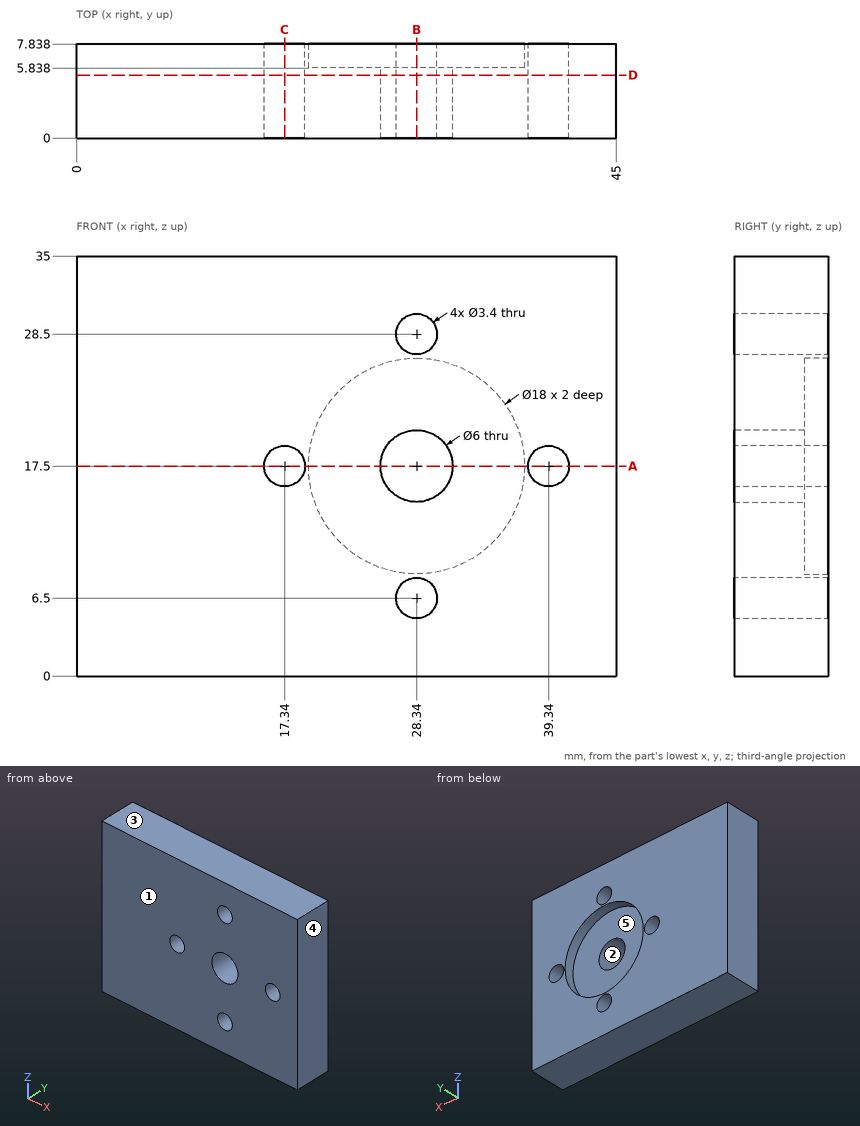
Geometry: see drawing. Coordinates: mm, zero at the bounding-box minimum. A direction names the side the tool comes from. Give positions to 0.01 mm unless a question says otherwise; leave off trailing zeros. Loops run counter-clockwise (first coordinate to the right, second up) from the corner with the lowest first, then second, coordinate; pieces in that order, holes last. Notation, with made-up numbers: (-17.75, -23) -> (-7.75, -23) arc R37 cw to (-7.75, 15) -> close; hole circle Ø3 at (-12, 40.5). An arc over 180 degrees is marked (long way). Put each result on its own line as item: value.
1. Cut plane B-B (x = 28.34). Return the cut outline in (y, z).
Taken from the geometry:
outline: (0, 0) -> (7.84, 0) -> (7.84, 4.8) -> (0, 4.8) -> close; (0, 8.2) -> (7.84, 8.2) -> (7.84, 8.5) -> (5.84, 8.5) -> (5.84, 14.5) -> (0, 14.5) -> close; (0, 20.5) -> (5.84, 20.5) -> (5.84, 26.5) -> (7.84, 26.5) -> (7.84, 26.8) -> (0, 26.8) -> close; (0, 30.2) -> (7.84, 30.2) -> (7.84, 35) -> (0, 35) -> close
2. Cut plane C-C (x = 17.34). Return the cut outline in (y, z), plus the area to 3 significant figures.
Taken from the geometry:
outline: (0, 0) -> (7.84, 0) -> (7.84, 15.8) -> (0, 15.8) -> close; (0, 19.2) -> (7.84, 19.2) -> (7.84, 35) -> (0, 35) -> close
area: 248 mm2
3. Cut plane A-A (z = 17.5). Return the cut outline in (x, y).
Taken from the geometry:
outline: (0, 0) -> (15.64, 0) -> (15.64, 7.84) -> (0, 7.84) -> close; (19.04, 0) -> (25.34, 0) -> (25.34, 5.84) -> (19.34, 5.84) -> (19.34, 7.84) -> (19.04, 7.84) -> close; (31.34, 0) -> (37.64, 0) -> (37.64, 7.84) -> (37.34, 7.84) -> (37.34, 5.84) -> (31.34, 5.84) -> close; (41.04, 0) -> (45, 0) -> (45, 7.84) -> (41.04, 7.84) -> close
4. Ray query, line 1 along X through (y, z) = (6, 17.5); line 2 along X through (y, z) = (3, 17.5); line 3 along X through (y, z) = (6.5, 6.5). Return the intervals inside material, ascending. Write a range as [from, to].
Taken from the geometry:
line 1: x = [0, 15.64], [19.04, 19.34], [37.34, 37.64], [41.04, 45]
line 2: x = [0, 15.64], [19.04, 25.34], [31.34, 37.64], [41.04, 45]
line 3: x = [0, 26.64], [30.04, 45]
5. Cut plane D-D (y = 5.25). Return the cut outline in (x, z), plus the area to 3 significant figures.
Taken from the geometry:
outline: (0, 0) -> (45, 0) -> (45, 35) -> (0, 35) -> close; hole circle Ø3.4 at (17.34, 17.5); hole circle Ø6 at (28.34, 17.5); hole circle Ø3.4 at (28.34, 6.5); hole circle Ø3.4 at (28.34, 28.5); hole circle Ø3.4 at (39.34, 17.5)
area: 1,510 mm2
6. Pull-direction query (Z, two-part tool) for the marked faces 1, 2 and 3; classes: released by +Z, released by -Z, zero draft, split by the parting line, or undercut.
Taken from the geometry:
face 1: zero draft
face 2: undercut
face 3: released by +Z
7. Set-up query: the marked faces 4 and 5. Return all of +Z, -Z, +X, -X, +Y, -Y with unobstructed straight access to the full face (end or side cutting, diameter ignored); none if empty.
Taken from the geometry:
face 4: +Z, -Z, +X, +Y, -Y
face 5: +Y
8. Pin query (flat end, axial travel): P1, Ø5.5, axis at x = 28.34, z = 6.5, coming from the +Y side; P2, Ø11, axis at x = 28.34, z = 17.5, coming from the +Y side. Return the tip coordinate at first contact, or that it passes through.
Taken from the geometry:
P1: stops at y = 7.84
P2: stops at y = 5.84
